Check sheet for the drawn part. Datum: minimum x, y, z corner. Units: mm. Round coordinates to 2 decimals unless told otherwise and drop trailing zeros. Write each loop counter-clockwise with the first axis right and the second up, starting at its lowest first coordinate (ties: lowest second). Pieces come first, ordered by that corner, then holes. Notation, with made-up numbers: M -33.75,70.5 L 22.25,70.5 A8 ccw 22.25,82.5 Z; hole C 79.5,31.5 d5. An arc over 180 degrees is marked long. Use a Markdown table: item, result.
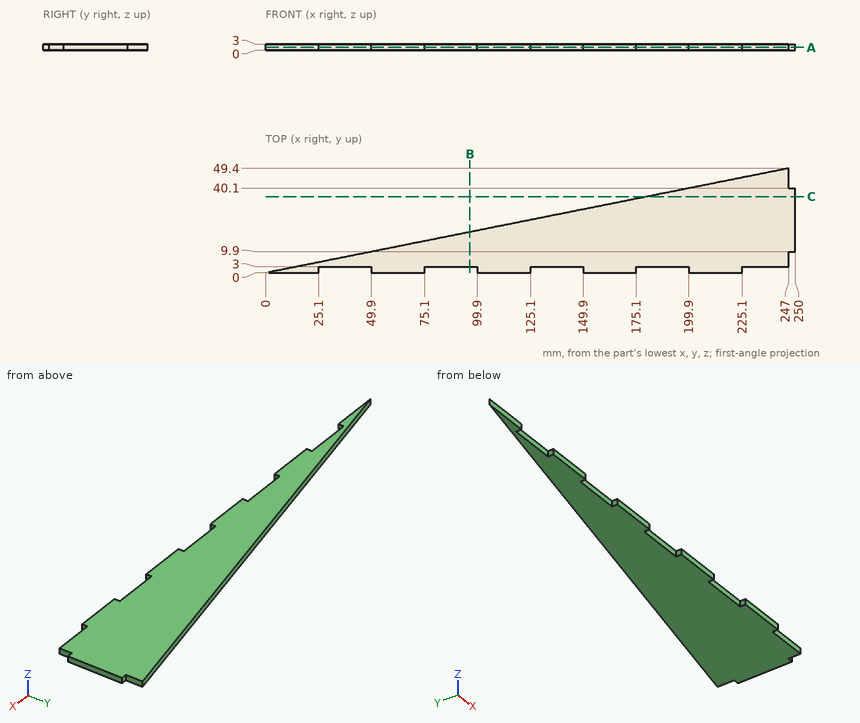
Item 1: Material ranges on line 1 along Y through (x, z) = (89, 2.3); line 2 along Y through (x, z) = (154, 2.3), recorded low to high. Write a range as from..to.
Outcome:
| item | result |
|---|---|
| line 1 | y = 3..17.8 |
| line 2 | y = 0..30.8 |
Item 2: Go/stop test with flat-tipped pins: pin 1 (0.9 mm diameter, centred on y = 2, z = 2, fed in from +X); pin 2 (1 mm diameter, centred on y = 7, z = 2, fed in from +X); pin 3 (1 mm diameter, centred on x = 182, z = 2, fed in from +Y). Record where each tip stops, or that it passes through.
Outcome:
| item | result |
|---|---|
| pin 1 | stops at x = 225.1 |
| pin 2 | stops at x = 247 |
| pin 3 | stops at y = 36.5 |
Item 3: Cross-section at A-A, the plane z = 1.35. Record the cut outline in (x, y), and give its area (3 significant figures).
Outcome:
| item | result |
|---|---|
| outline | M 0,0 L 25.1,0 L 25.1,3 L 49.9,3 L 49.9,0 L 75.1,0 L 75.1,3 L 99.9,3 L 99.9,0 L 125.1,0 L 125.1,3 L 149.9,3 L 149.9,0 L 175.1,0 L 175.1,3 L 199.9,3 L 199.9,0 L 225.1,0 L 225.1,3 L 247,3 L 247,9.9 L 250,9.9 L 250,40.1 L 247,40.1 L 247,49.4 Z |
| area | 5,830 mm2 |
Item 4: Cross-section at B-B, the plane x = 96.5. Record the cut outline in (y, z), and give its area (3 significant figures).
Outcome:
| item | result |
|---|---|
| outline | M 3,0 L 19.3,0 L 19.3,3 L 3,3 Z |
| area | 48.9 mm2 |
Item 5: Cross-section at C-C, the plane y = 36. Record the cut outline in (x, z).
Outcome:
| item | result |
|---|---|
| outline | M 180,0 L 250,0 L 250,3 L 180,3 Z |
